Verification items for the finished model (mm, model axes). A direction names the side the tool comes from. Give positions to 0.01 mm unless a question says otherwise; leave off trailing zeros. Loops run counter-clockwise (first coordinate to the right, second up) from the corner with the lowest first, then second, coordinate; pieces in that order, holes last. Notation, with made-up numbers: (62.5, 39) -> (88.5, 39) arc R16 ccw to (88.5, 53) -> close; hole circle Ø4 at (72, -39). An arc over 180 degrees is marked (long way). Answer in a Markdown table with one row per item. Add a question column.
Q1. Section check C-C on x = -19. Enter the section's corners in (y, z).
Q2. Release check for a two-part mould opening along Y. For faces 6 (the face through (0, -10, -55)), 7 (the face through (44.93, -7.31, 1.76)), 8 (the face through (53, -1, 1)) record: pulls with the +Y half, pulls with the -Y half, needs draft (parallel to the pull), parting line crosses it, or undercut.
Q3. Set-up check for faces 1 (the face through (-1, 2, -1)), 2 (the face through (-45.07, -7.52, 1.76)), 3 (the face through (-17.017, 1.014, 18.24)), 4 (the face through (45, -26, 40)), 5 (the face through (-47, -4, -25)): record each of +Z, -Z, +X, -X, +Y, -Y from which the full face is reachable in a straight line by a thin tool's end or side.
Q4. Gauge pin test, flat ends, axial feed: P1, Ø5, axis at x = 43, z = -25, coming from the -Y side; P2, Ø1.5, axis at x = 10, z = -8, coming from the -Y side; P3, Ø13.5, axis at x = -21, y = -15.5, coming from the +Z side. Record the tip position at first contact, or that the pin passes through.
Q5. Section check D-D on z = -40. Give the number of separate pieces and of enclosed holes in the cut face, and give its area (3 significant figures).
Q6. Section check A-A on x = 0. Enter the section's corners in (y, z), and give its area (3 significant figures).
Q7. Material ranges on probe 1 along X at (y, z) = (1.5, -40); probe 2 along Z at (x, y) = (-21, -7); probe 3 along X at (y, z) = (-6, -40), recorded low to high.
```python
from build123d import *
from build123d.topology import SkipClean

# Parameters (mm, degrees)
SKETCH1_W           = 110
SKETCH1_H           = 110
BOSS_EXTRUDE1_DEPTH = 2
SKETCH2_R           = 2
CUT_EXTRUDE1_DEPTH  = 78.807454656
SKETCH3_W           = 5
SKETCH3_H           = 110
BOSS_EXTRUDE2_DEPTH = 32
SKETCH4_R           = 1.5
CUT_EXTRUDE2_DEPTH  = 85.888161719
SKETCH5_R           = 2
CUT_EXTRUDE3_DEPTH  = 85.107074613
CHAMFER1_SIZE       = 14.825609685
CHAMFER1_SIZE_2     = 10
SKETCH6_R           = 4
CUT_EXTRUDE4_DEPTH  = 85.107074613
CHAMFER2_SIZE       = 5
BOSS_EXTRUDE3_DEPTH = 2
CUT_EXTRUDE5_DEPTH  = 2
CHAMFER3_SIZE       = 5
CUT_EXTRUDE6_DEPTH  = 2
BOSS_EXTRUDE4_DEPTH = 108
SKETCH12_R          = 2
CUT_EXTRUDE7_DEPTH  = 85.107074613
SKETCH13_R          = 4
CUT_EXTRUDE8_DEPTH  = 25


# Some blends are built 0.0001 mm under size
with BuildPart() as part:
    # Sketch1 → Boss-Extrude1 (new body)
    with BuildSketch(Plane(origin=(0, 0, 0), x_dir=(1, 0, 0), z_dir=(0, 1, 0))):
        Rectangle(SKETCH1_W, SKETCH1_H)
    extrude(amount=BOSS_EXTRUDE1_DEPTH)

    # Sketch2 → Cut-Extrude1 (cut, through all)
    with BuildSketch(Plane(origin=(0, 2, 0), x_dir=(1, 0, 0), z_dir=(0, 1, 0))):
        with Locations(Location((-43, -40, 0), (0, 0, 270))):
            Circle(SKETCH2_R)
        with Locations(Location((-43, -27.5, 0), (0, 0, 270))):
            Circle(SKETCH2_R)
        with Locations(Location((-19, -18.5, 0), (0, 0, 270))):
            Circle(SKETCH2_R)
    extrude(amount=-CUT_EXTRUDE1_DEPTH, mode=Mode.SUBTRACT)

    # Sketch3 → Boss-Extrude2 (add)
    with BuildSketch(Plane.XZ):
        with Locations((-52.5, 0)):
            Rectangle(SKETCH3_W, SKETCH3_H)
        with Locations((52.5, 0)):
            Rectangle(SKETCH3_W, SKETCH3_H)
    extrude(amount=BOSS_EXTRUDE2_DEPTH)

    # Sketch4 → Cut-Extrude2 (cut, through all)
    with BuildSketch(Plane(origin=(0, 2, 0), x_dir=(1, 0, 0), z_dir=(0, 1, 0))):
        with Locations(Location((0, 30, 0), (0, 0, 270))):
            Circle(SKETCH4_R)
        with Locations(Location((0, -20, 0), (0, 0, 270))):
            Circle(SKETCH4_R)
    extrude(amount=-CUT_EXTRUDE2_DEPTH, mode=Mode.SUBTRACT)

    # Sketch5 → Cut-Extrude3 (cut, through all)
    with BuildSketch(Plane.XZ):
        with Locations(Location((-43, -25, 0), (0, 0, 270))):
            Circle(SKETCH5_R)
        with Locations(Location((-43, -40, 0), (0, 0, 270))):
            Circle(SKETCH5_R)
        with Locations(Location((43, -25, 0), (0, 0, 270))):
            Circle(SKETCH5_R)
        with Locations(Location((43, -40, 0), (0, 0, 270))):
            Circle(SKETCH5_R)
    extrude(amount=-CUT_EXTRUDE3_DEPTH, mode=Mode.SUBTRACT)

    # Chamfer1
    # the kernel refuses this chamfer: 14.825609685, 10 mm, written as the material it adds along each edge
    with BuildSketch(Plane(origin=(-50, 0, 55), x_dir=(-0.021644705014774085, -0.9997657259302418, 0), z_dir=(0, 0, -1))) as chamfer1_piece_1_section:
        Polygon((CHAMFER1_SIZE * 0.999765725939, -CHAMFER1_SIZE * 0.021644705015), (-CHAMFER1_SIZE_2 * 0.0216447050148, -CHAMFER1_SIZE_2 * 0.99976572593), (0, 0), align=None)
    chamfer1_piece_1 = extrude(amount=110, mode=Mode.PRIVATE)
    chamfer1_piece_1 = chamfer1_piece_1 - Plane(origin=(-43, -5.019728398, 40), x_dir=(0, 0, 1), z_dir=(0, 1, 0)) * Cylinder(2, 280, mode=Mode.PRIVATE)
    chamfer1_piece_1 = chamfer1_piece_1 - Plane(origin=(-43, -5.019728398, 27.5), x_dir=(0, 0, 1), z_dir=(0, 1, 0)) * Cylinder(2, 280, mode=Mode.PRIVATE)
    chamfer1_piece_1 = chamfer1_piece_1 - Plane(origin=(-43, -5.019728398, -25), x_dir=(0, 0, -1), z_dir=(0, -1, 0)) * Cylinder(2, 280, mode=Mode.PRIVATE)
    chamfer1_piece_1 = chamfer1_piece_1 - Plane(origin=(-43, -5.019728398, -40), x_dir=(0, 0, -1), z_dir=(0, -1, 0)) * Cylinder(2, 280, mode=Mode.PRIVATE)
    add(chamfer1_piece_1)
    with BuildSketch(Plane(origin=(50, 0, 55), x_dir=(-0.9988697089125116, 0.04753214298802855, 0), z_dir=(0, 0, -1))) as chamfer1_piece_2_section:
        Polygon((CHAMFER1_SIZE_2 * 0.998869708913, -CHAMFER1_SIZE_2 * 0.047532142988), (-CHAMFER1_SIZE * 0.0475321429884, -CHAMFER1_SIZE * 0.998869708921), (0, 0), align=None)
    chamfer1_piece_2 = extrude(amount=110, mode=Mode.PRIVATE)
    chamfer1_piece_2 = chamfer1_piece_2 - Plane(origin=(43, -4.982049295, -25), x_dir=(0, 0, -1), z_dir=(0, -1, 0)) * Cylinder(2, 280, mode=Mode.PRIVATE)
    chamfer1_piece_2 = chamfer1_piece_2 - Plane(origin=(43, -4.982049295, -40), x_dir=(0, 0, -1), z_dir=(0, -1, 0)) * Cylinder(2, 280, mode=Mode.PRIVATE)
    add(chamfer1_piece_2)

    # Sketch6 → Cut-Extrude4 (cut, through all)
    with BuildSketch(Plane.XZ):
        with Locations((-43, 40)):
            Circle(SKETCH6_R)
        with Locations((-43, 27.5)):
            Circle(SKETCH6_R)
        with Locations((-43, -25)):
            Circle(SKETCH6_R)
        with Locations((-43, -40)):
            Circle(SKETCH6_R)
        with Locations((43, -25)):
            Circle(SKETCH6_R)
        with Locations((43, -40)):
            Circle(SKETCH6_R)
    extrude(amount=CUT_EXTRUDE4_DEPTH, mode=Mode.SUBTRACT)

    # Chamfer2
    chamfer2_edges = [part.edges().sort_by_distance(p)[0] for p in [
        (55, 2, 0),
        (-55, 2, 0),
    ]]
    chamfer(chamfer2_edges, length=CHAMFER2_SIZE)

    # Sketch8 → Boss-Extrude3 (add)
    with BuildSketch(Plane(origin=(0, 0, -55), x_dir=(-1, 0, 0), z_dir=(0, 0, -1))):
        Polygon((-55, -32), (55, -32), (55, -3), (50, 2), (-50, 2), (-55, -3), align=None)
    extrude(amount=-BOSS_EXTRUDE3_DEPTH)

    # Sketch9 → Cut-Extrude5 (cut)
    with BuildSketch(Plane(origin=(0, 0, -55), x_dir=(-1, 0, 0), z_dir=(0, 0, -1))):
        with BuildLine():
            Line((-31.125, -8), (-31.125, -20))
            ThreePointArc((-31.125, -20), (-33.375, -22.25), (-35.625, -20))
            Line((-35.625, -20), (-35.625, -8))
            ThreePointArc((-35.625, -8), (-33.375, -5.75), (-31.125, -8))
        make_face()
    cut_extrude5 = extrude(amount=-CUT_EXTRUDE5_DEPTH, mode=Mode.SUBTRACT)

    # Mirror1: Cut-Extrude5 across plane
    add(cut_extrude5.mirror(Plane(origin=(0, 0, 0), x_dir=(0, 0, 1), z_dir=(1, 0, 0))), mode=Mode.SUBTRACT)

    # Chamfer3
    chamfer3_edges = [part.edges().sort_by_distance(p)[0] for p in [
        (50, -32, 1),
        (-50, -32, 1),
    ]]
    chamfer(chamfer3_edges, length=CHAMFER3_SIZE - 0.0001)  # a hair under: the kernel refuses the full size

    # Sketch10 → Cut-Extrude6 (cut)
    with SkipClean():  # the faces are left unmerged after this step: merging them gives an invalid solid
        with BuildSketch(Plane.XY.offset(-53)):
            Polygon((-50, -27), (50, -27), (55, -32), (-55, -32), align=None)
        extrude(amount=-CUT_EXTRUDE6_DEPTH, mode=Mode.SUBTRACT)

    # Sketch11 → Boss-Extrude4 (add)
    with SkipClean():  # the faces are left unmerged after this step: merging them gives an invalid solid
        with BuildSketch(Plane.XY.offset(55)):
            Polygon((-50, -14.825609685), (-37.825609685, -27), (-50, -27), align=None)
        boss_extrude4 = extrude(amount=-BOSS_EXTRUDE4_DEPTH)

    # Sketch12 → Cut-Extrude7 (cut, through all)
    with SkipClean():  # the faces are left unmerged after this step: merging them gives an invalid solid
        with BuildSketch(Plane(origin=(0, 0, 0), x_dir=(1, 0, 0), z_dir=(0, 1, 0))):
            with Locations(Location((-43, -40, 0), (0, 0, 270))):
                Circle(SKETCH12_R)
            with Locations(Location((-43, -27.5, 0), (0, 0, 270))):
                Circle(SKETCH12_R)
            with Locations(Location((-43, 25, 0), (0, 0, 90))):
                Circle(SKETCH12_R)
            with Locations(Location((-43, 40, 0), (0, 0, 90))):
                Circle(SKETCH12_R)
        cut_extrude7 = extrude(amount=-CUT_EXTRUDE7_DEPTH, mode=Mode.SUBTRACT)

    # Sketch13 → Cut-Extrude8 (cut)
    with SkipClean():  # the faces are left unmerged after this step: merging them gives an invalid solid
        with BuildSketch(Plane.XZ):
            with Locations((-43, 40)):
                Circle(SKETCH13_R)
            with Locations((-43, 27.5)):
                Circle(SKETCH13_R)
            with Locations((-43, -25)):
                Circle(SKETCH13_R)
            with Locations((-43, -40)):
                Circle(SKETCH13_R)
        cut_extrude8 = extrude(amount=CUT_EXTRUDE8_DEPTH, mode=Mode.SUBTRACT)

    # Mirror2: Boss-Extrude4, Cut-Extrude7, Cut-Extrude8 across plane
    with SkipClean():  # the faces are left unmerged after this step: merging them gives an invalid solid
        add(boss_extrude4.mirror(Plane(origin=(0, 0, 0), x_dir=(0, 0, 1), z_dir=(1, 0, 0))))
        add(cut_extrude7.mirror(Plane(origin=(0, 0, 0), x_dir=(0, 0, 1), z_dir=(1, 0, 0))), mode=Mode.SUBTRACT)
        add(cut_extrude8.mirror(Plane(origin=(0, 0, 0), x_dir=(0, 0, 1), z_dir=(1, 0, 0))), mode=Mode.SUBTRACT)


solid = part.part
```
Taken from the geometry:
| question | item | result |
|---|---|---|
| 1 | outline | (-27, -55) -> (2, -55) -> (2, 16.5) -> (0, 16.5) -> (0, -53) -> (-27, -53) -> close; (0, 20.5) -> (2, 20.5) -> (2, 55) -> (0, 55) -> close |
| 2 | face 6 | needs draft |
| 2 | face 7 | undercut |
| 2 | face 8 | pulls with the +Y half |
| 3 | face 1 | +Z, -Z, +X, -X, +Y |
| 3 | face 2 | +Z |
| 3 | face 3 | +Y, -Y |
| 3 | face 4 | -Y |
| 3 | face 5 | none |
| 4 | P1 | stops at y = -27 |
| 4 | P2 | stops at y = 0 |
| 4 | P3 | stops at z = -53 |
| 5 | separate pieces | 5 |
| 5 | enclosed holes | 0 |
| 5 | area | 630 mm² |
| 6 | outline | (-27, -55) -> (2, -55) -> (2, -31.5) -> (0, -31.5) -> (0, -53) -> (-27, -53) -> close; (0, -28.5) -> (2, -28.5) -> (2, 18.5) -> (0, 18.5) -> close; (0, 21.5) -> (2, 21.5) -> (2, 55) -> (0, 55) -> close |
| 6 | area | 262 mm² |
| 7 | probe 1 | x = -50.5 to -45, -41 to 41, 45 to 50.5 |
| 7 | probe 2 | z = -55 to -53 |
| 7 | probe 3 | x = -55 to -47, 47 to 55 |
